For this review, use the dimensioned drawing (mm, ordinates from the lowest corner) and the shaded views. Give positions to 0.01 mm unless a question says otherwise; leave off trailing zeros. Loops run counter-clockwise (first coordinate to the right, second up) from the corner with the lowest first, then second, coordinate; pieces in that order, holes last. Notation, with made-up numbers: (37.5, 19) - (53.5, 19) arc R18 cw to (53.5, 53) - close; hole circle Ø2 at (-22, 21). An arc over 180 degrees is marked (long way). Write each question's results on one line, items separated by ' | '.
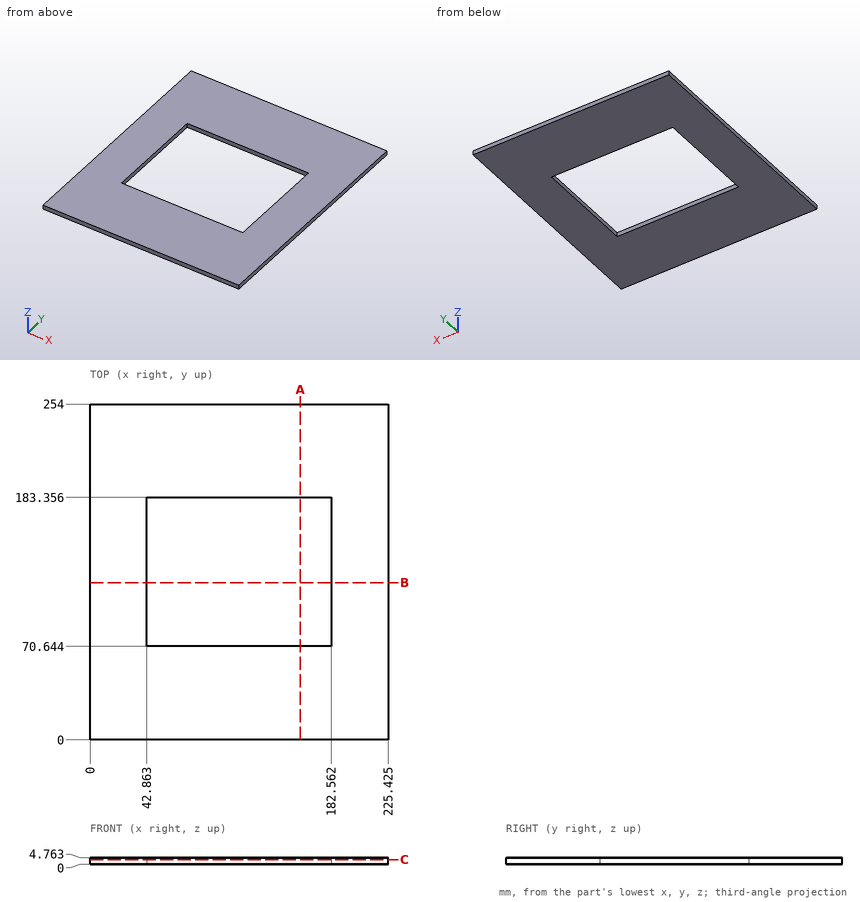
Item 1: Wall thickness on probe 1 along Y at (x, z) = (64, 2.05); probe 2 along X at (y, z) = (71, 1.2) (1 decimal): over which ranges is each line inside the solid? List them lowest first.
Output values:
probe 1: y = 0 to 70.64, 183.36 to 254 | probe 2: x = 0 to 42.9, 182.6 to 225.4
Item 2: We need section C-C on z = 3.45. Give the boundary of the cut face in (x, y) (1 decimal), then the cut area to 3 significant figures.
Output values:
outline: (0, 0) - (225.4, 0) - (225.4, 254) - (0, 254) - close; hole (42.9, 70.6) - (182.6, 70.6) - (182.6, 183.4) - (42.9, 183.4) - close | area: 41,500 mm²
Item 3: We need section B-B on y = 119. Give the boundary of the cut face in (x, z) (1 decimal), then the cut area to 3 significant figures.
Output values:
outline: (0, 0) - (42.9, 0) - (42.9, 4.8) - (0, 4.8) - close; (182.6, 0) - (225.4, 0) - (225.4, 4.8) - (182.6, 4.8) - close | area: 408 mm²
Item 4: We need section A-A on x = 159. Give the boundary of the cut face in (y, z).
Output values:
outline: (0, 0) - (70.64, 0) - (70.64, 4.76) - (0, 4.76) - close; (183.36, 0) - (254, 0) - (254, 4.76) - (183.36, 4.76) - close
